Source: CAD feature listing. Evaluate the final solid. Frame: model axes, mm. Face numbers are marked on the shaded views. A direction names the side the tool comes from. Round coordinates to 2 decimals unless told otherwise and drop trailing zeros. Order: outer loops, then holes, each group sorted by start corner. A loop starts at its lowest first (then second) coordinate and runs counter-clockwise, first axis right, second up. Notation, with made-up numbers: (80, -10.75) - (88, -10.75) arc R30 cw to (88, 13.25) - close; hole circle Ø10 at (-27.75, 6). An arc over 180 degrees is marked (long way). Return JSON: item names as keys, results as strings. Group by question number.
1) Ray query, line 1 (X direction, y = 346, z = -62.5); line 2 (Z direction, x = 178, y = 336.5); line 3 (Z direction, x = 109, y = -21.5). Return the intervals inside material, ascending. Write a range as from..to.
2) Section A-A, the plane z = -836. Return loops of the section in (x, y), plus the area to 3 significant figures.
3) Section B-B, the plane x = 41. Return loops of the section in (y, z), plus the area to 3 significant figures.
4) Mould query, pull axis Z, two halves, no side actions, for the marked faces 5, 6, 7 and 8. Classes: pulls with the +Z half, pulls with the -Z half, needs draft (parallel to the pull), parting line crosses it, or undercut.
5) Section C-C, the plane x = 172. Return loops of the section in (y, z), plus the area to 3 significant figures.
6) Contact query for flat-ended pins moving along their axis: P1, Ø8, axis at x = 75.5, z = -356, coming from the +Y side; P2, Ø6, axis at x = 497, z = -359, coming from the -Y side. Output: stop coordinate, or through.
7) Access query for the marked faces 1, 2, 3 and 4. Directions: +Z, -Z, +X, -X, +Y, -Y. A direction counts if a zero-diameter tool reaches every point of the face in a straight line with its end or side. Return the directions, or none.
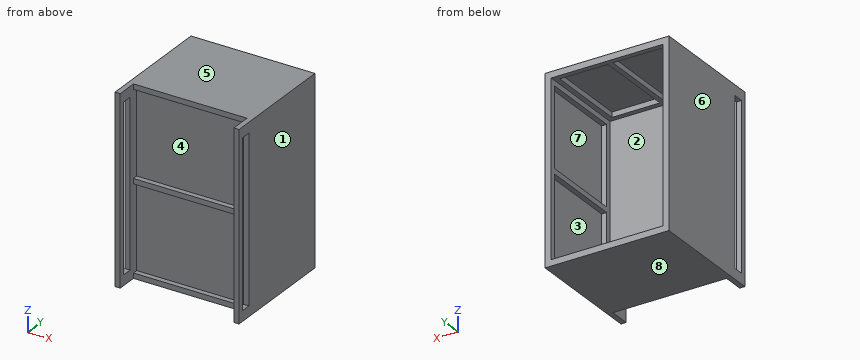
```python
from build123d import *

# Parameters (mm, degrees)
SKETCH1_W            = 609.6
SKETCH1_H            = 457.2
BOSS_EXTRUDE1_DEPTH  = 5
SKETCH2_W            = 5
SKETCH2_H            = 914.4
BOSS_EXTRUDE2_DEPTH  = 457.2
SKETCH3_W            = 609.6
SKETCH3_H            = 457.2
BOSS_EXTRUDE3_DEPTH  = 5
SKETCH4_W            = 914.4
SKETCH4_H            = 457.2
BOSS_EXTRUDE4_DEPTH  = 5
SKETCH5_W            = 609.6
SKETCH5_H            = 914.4
BOSS_EXTRUDE5_DEPTH  = 5
SKETCH6_W            = 609.6
SKETCH6_H            = 914.4
SKETCH6_W_2          = 558.8
SKETCH6_H_2          = 863.6
BOSS_EXTRUDE6_DEPTH  = 25.4
SKETCH7_W            = 25.4
SKETCH7_H            = 863.6
BOSS_EXTRUDE7_DEPTH  = 25.4
SKETCH10_W           = 904.4
SKETCH10_H           = 452.2
SKETCH10_W_2         = 853.6
SKETCH10_H_2         = 401.4
BOSS_EXTRUDE8_DEPTH  = 25.4
SKETCH22_W           = 548.8
SKETCH22_H           = 452.2
SKETCH22_W_2         = 236.3
SKETCH22_H_2         = 401.4
BOSS_EXTRUDE14_DEPTH = 25.4
SKETCH15_W           = 25.4
SKETCH15_H           = 401.4
BOSS_EXTRUDE15_DEPTH = 25.4
SKETCH23_W           = 25.4
SKETCH23_H           = 401.4
BOSS_EXTRUDE16_DEPTH = 25.4
SKETCH17_W           = 914.4
SKETCH17_H           = 101.6
SKETCH17_W_2         = 812.8
SKETCH17_H_2         = 50.8
BOSS_EXTRUDE17_DEPTH = 25.4
SKETCH25_W           = 25.4
SKETCH25_H           = 863.6
CUT_EXTRUDE1_DEPTH   = 25.4
SKETCH26_W           = 558.8
SKETCH26_H           = 25.4
BOSS_EXTRUDE18_DEPTH = 25.4


with BuildPart() as part:
    # Sketch1 → Boss-Extrude1 (new body)
    with BuildSketch(Plane.XY):
        with Locations((304.8, 228.6)):
            Rectangle(SKETCH1_W, SKETCH1_H)
    extrude(amount=BOSS_EXTRUDE1_DEPTH)

    # Sketch2 → Boss-Extrude2 (add)
    with BuildSketch(Plane(origin=(0, 0, 0), x_dir=(1, 0, 0), z_dir=(0, 1, 0))):
        with Locations((2.5, 452.2)):
            Rectangle(SKETCH2_W, SKETCH2_H)
    extrude(amount=BOSS_EXTRUDE2_DEPTH)

    # Sketch3 → Boss-Extrude3 (add)
    with BuildSketch(Plane(origin=(0, 0, -909.4), x_dir=(-1, 0, 0), z_dir=(0, 0, -1))):
        with Locations((-304.8, 228.6)):
            Rectangle(SKETCH3_W, SKETCH3_H)
    extrude(amount=-BOSS_EXTRUDE3_DEPTH)

    # Sketch4 → Boss-Extrude4 (add)
    with BuildSketch(Plane(origin=(609.6, 0, 0), x_dir=(0, 0, -1), z_dir=(1, 0, 0))):
        with Locations((452.2, 228.6)):
            Rectangle(SKETCH4_W, SKETCH4_H)
    extrude(amount=-BOSS_EXTRUDE4_DEPTH)

    # Sketch5 → Boss-Extrude5 (add)
    with BuildSketch(Plane(origin=(0, 0, 0), x_dir=(-1, 0, 0), z_dir=(0, -1, 0))):
        with Locations((-304.8, 452.2)):
            Rectangle(SKETCH5_W, SKETCH5_H)
    extrude(amount=-BOSS_EXTRUDE5_DEPTH)

    # Sketch6 → Boss-Extrude6 (add)
    with BuildSketch(Plane.XZ):
        with Locations((304.8, -452.2)):
            Rectangle(SKETCH6_W, SKETCH6_H)
        with Locations((304.8, -452.2)):
            Rectangle(SKETCH6_W_2, SKETCH6_H_2, mode=Mode.SUBTRACT)
    extrude(amount=BOSS_EXTRUDE6_DEPTH)

    # Sketch7 → Boss-Extrude7 (add)
    with BuildSketch(Plane.XZ):
        with Locations((304.8, -452.2)):
            Rectangle(SKETCH7_W, SKETCH7_H)
    extrude(amount=BOSS_EXTRUDE7_DEPTH)

    # Sketch10 → Boss-Extrude8 (add)
    with BuildSketch(Plane.ZY.offset(-604.6)):
        with Locations((-452.2, 231.1)):
            Rectangle(SKETCH10_W, SKETCH10_H)
        with Locations((-452.2, 231.1)):
            Rectangle(SKETCH10_W_2, SKETCH10_H_2, mode=Mode.SUBTRACT)
    extrude(amount=BOSS_EXTRUDE8_DEPTH)


with BuildPart() as body_2:
    # Mirror3: mirrored copy
    add(part.part.mirror(Plane(origin=(304.8, 457.2, -904.4), x_dir=(0, 0, 1), z_dir=(1, 0, 0))))


with BuildPart() as part_1:
    add(part.part)

    add(body_2.part)  # Boss-Extrude14 merges body 2
    # Sketch22 → Boss-Extrude14 (add)
    with BuildSketch(Plane.XY.offset(-904.4)):
        with Locations((304.8, 231.1)):
            Rectangle(SKETCH22_W, SKETCH22_H)
        with Locations((173.95, 231.1)):
            Rectangle(SKETCH22_W_2, SKETCH22_H_2, mode=Mode.SUBTRACT)
        with Locations((435.65, 231.1)):
            Rectangle(SKETCH22_W_2, SKETCH22_H_2, mode=Mode.SUBTRACT)
    extrude(amount=BOSS_EXTRUDE14_DEPTH)

    # Sketch15 → Boss-Extrude15 (add)
    with BuildSketch(Plane(origin=(5, 0, 0), x_dir=(0, 0, -1), z_dir=(1, 0, 0))):
        with Locations((38.1, 231.1)):
            Rectangle(SKETCH15_W, SKETCH15_H)
        with Locations((866.3, 231.1)):
            Rectangle(SKETCH15_W, SKETCH15_H)
        with Locations((452.2, 231.1)):
            Rectangle(SKETCH15_W, SKETCH15_H)
    extrude(amount=BOSS_EXTRUDE15_DEPTH)

    # Sketch23 → Boss-Extrude16 (add)
    with BuildSketch(Plane.ZY.offset(-604.6)):
        with Locations((-38.1, 231.1)):
            Rectangle(SKETCH23_W, SKETCH23_H)
        with Locations((-452.2, 231.1)):
            Rectangle(SKETCH23_W, SKETCH23_H)
        with Locations((-866.3, 231.1)):
            Rectangle(SKETCH23_W, SKETCH23_H)
    extrude(amount=BOSS_EXTRUDE16_DEPTH)

    # Mirror9: part across plane


with BuildPart() as part_2:
    add(part_1.part)
    add(part_1.part.mirror(Plane.XY.offset(-452.2)))

    # Sketch17 → Boss-Extrude17 (add)
    with BuildSketch(Plane(origin=(0, 0, 5), x_dir=(0, 0, -1), z_dir=(1, 0, 0))):
        with Locations((457.2, -76.2)):
            Rectangle(SKETCH17_W, SKETCH17_H)
        with Locations((457.2, -76.2)):
            Rectangle(SKETCH17_W_2, SKETCH17_H_2, mode=Mode.SUBTRACT)
    extrude(amount=BOSS_EXTRUDE17_DEPTH)

    # Mirror10: part across plane


with BuildPart() as part_3:
    add(part_2.part)
    add(part_2.part.mirror(Plane(origin=(304.8, 457.2, -904.4), x_dir=(0, 0, 1), z_dir=(1, 0, 0))))

    # Sketch25 → Cut-Extrude1 (cut)
    with BuildSketch(Plane.XZ.offset(25.4)):
        with Locations((304.8, -452.2)):
            Rectangle(SKETCH25_W, SKETCH25_H)
    extrude(amount=-CUT_EXTRUDE1_DEPTH, mode=Mode.SUBTRACT)

    # Sketch26 → Boss-Extrude18 (add)
    with BuildSketch(Plane.XZ):
        with Locations((304.8, -452.2)):
            Rectangle(SKETCH26_W, SKETCH26_H)
    extrude(amount=BOSS_EXTRUDE18_DEPTH)


solid = part_3.part
```
Geometry check:
{
 "1": {"line 1": "0..5, 604.6..609.6", "line 2": "-909.4..-904.4, 0..5", "line 3": "-909.4..-884, -464.9..-439.5, -20.4..5"},
 "2": {"outline": "(0, -127) - (25.4, -127) - (25.4, -101.6) - (0, -101.6) - close; (0, -50.8) - (25.4, -50.8) - (25.4, 0) - (584.2, 0) - (584.2, -50.8) - (609.6, -50.8) - (609.6, 457.2) - (579.2, 457.2) - (579.2, 431.8) - (604.6, 431.8) - (604.6, 30.4) - (579.2, 30.4) - (579.2, 5) - (30.4, 5) - (30.4, 30.4) - (5, 30.4) - (5, 431.8) - (30.4, 431.8) - (30.4, 457.2) - (0, 457.2) - close; (584.2, -127) - (609.6, -127) - (609.6, -101.6) - (584.2, -101.6) - close", "area": "14,000 mm2"},
 "3": {"outline": "(-25.4, -909.4) - (457.2, -909.4) - (457.2, -879) - (5, -879) - (5, -25.4) - (457.2, -25.4) - (457.2, 5) - (-25.4, 5) - (-25.4, -20.4) - (0, -20.4) - (0, -439.5) - (-25.4, -439.5) - (-25.4, -464.9) - (0, -464.9) - (0, -884) - (-25.4, -884) - close", "area": "34,000 mm2"},
 "4": {"face 5": "pulls with the +Z half", "face 6": "needs draft", "face 7": "undercut", "face 8": "pulls with the -Z half"},
 "5": {"outline": "(-25.4, -909.4) - (457.2, -909.4) - (457.2, -879) - (431.8, -879) - (431.8, -904.4) - (30.4, -904.4) - (30.4, -879) - (5, -879) - (5, -25.4) - (30.4, -25.4) - (30.4, 0) - (431.8, 0) - (431.8, -25.4) - (457.2, -25.4) - (457.2, 5) - (-25.4, 5) - (-25.4, -20.4) - (0, -20.4) - (0, -439.5) - (-25.4, -439.5) - (-25.4, -464.9) - (0, -464.9) - (0, -884) - (-25.4, -884) - close", "area": "13,600 mm2"},
 "6": {"P1": "y = 5", "P2": "y = 0"},
 "7": {"face 1": "+Z, -Z, +X, +Y, -Y", "face 2": "+Y", "face 3": "none", "face 4": "-Y"}
}
